from build123d import *

# Parameters (mm, degrees)
SKETCH_2_R          = 10
EXTRUDE_1_DEPTH     = 30
EXTRUDE_START       = -10
EXTRUDE_2_DEPTH     = 10
CUT_EXTRUDE_4_DEPTH = 41.372064023
CUT_EXTRUDE_5_DEPTH = 41.372064023
CUT_EXTRUDE_6_DEPTH = 41.372064023
CUT_EXTRUDE_7_DEPTH = 41.372064023
SKETCH_10_R         = 5.05
CUT_EXTRUDE_8_DEPTH = 25
EXTRUDE_3_DEPTH     = 45
SKETCH_12_R         = 1
CUT_EXTRUDE_9_DEPTH = 79.386948681


with BuildPart() as part:
    # Sketch 2 → Extrude 1 (new body)
    with BuildSketch(Plane(origin=(0, 0, 0), x_dir=(1, 0, 0), z_dir=(0, 1, 0))):
        with Locations(Location((0, 0, 0), (0, 0, 270))):
            Circle(SKETCH_2_R)
    extrude(amount=EXTRUDE_1_DEPTH)

    # Sketch 4 → Extrude 2 (add)
    with BuildSketch(Plane(origin=(0, 30, 0), x_dir=(1, 0, 0), z_dir=(0, 1, 0)).offset(EXTRUDE_START)):
        with BuildLine():
            Line((7.857286278, -21.821134908), (4.965257474, -8.680219941))
            ThreePointArc((4.965257474, -8.680219941), (2.18360644, -9.758681413), (-0.792400015, -9.968555674))
            Line((-0.792400015, -9.968555674), (2.095178486, -23.089249172))
            Line((2.095178486, -23.089249172), (7.857286278, -21.821134908))
        make_face()
    extrude(amount=EXTRUDE_2_DEPTH)

    # Sketch 6 → Cut-Extrude 4 (cut, through all)
    with BuildSketch(Plane(origin=(2.913802079, 0, -0.641264293), x_dir=(-0.2149346210056599, 0, -0.9766284394247146), z_dir=(0.9766284394247146, 0, -0.2149346210056599))):
        with BuildLine():
            Line((-22.999943781, 25.008760147), (-22.999943781, 20))
            Line((-22.999943781, 20), (-18.179619595, 20))
            ThreePointArc((-18.179619595, 20), (-21.599118817, 21.533015498), (-22.999943781, 25.008760147))
        make_face()
    extrude(amount=-CUT_EXTRUDE_4_DEPTH, mode=Mode.SUBTRACT)

    # Sketch 6_3 → Cut-Extrude 5 (cut, through all)
    with BuildSketch(Plane(origin=(2.913802079, 0, -0.641264293), x_dir=(-0.2149346210056599, 0, -0.9766284394247146), z_dir=(0.9766284394247146, 0, -0.2149346210056599))):
        with BuildLine():
            Line((-22.999943781, 30), (-22.999943781, 25.008760147))
            ThreePointArc((-22.999943781, 25.008760147), (-21.691086809, 28.386338596), (-18.448057419, 30))
            Line((-18.448057419, 30), (-22.999943781, 30))
        make_face()
    extrude(amount=-CUT_EXTRUDE_5_DEPTH, mode=Mode.SUBTRACT)

    # Sketch 6_4 → Cut-Extrude 6 (cut, through all)
    with BuildSketch(Plane(origin=(2.913802079, 0, -0.641264293), x_dir=(-0.2149346210056599, 0, -0.9766284394247146), z_dir=(0.9766284394247146, 0, -0.2149346210056599))):
        with BuildLine():
            Line((-15.437501839, 25.006114345), (-20.537499094, 25.01140595))
            ThreePointArc((-20.537499094, 25.01140595), (-17.990146269, 22.45876152), (-15.437501839, 25.006114345))
        make_face()
    extrude(amount=-CUT_EXTRUDE_6_DEPTH, mode=Mode.SUBTRACT)

    # Sketch 6_5 → Cut-Extrude 7 (cut, through all)
    with BuildSketch(Plane(origin=(2.913802079, 0, -0.641264293), x_dir=(-0.2149346210056599, 0, -0.9766284394247146), z_dir=(0.9766284394247146, 0, -0.2149346210056599))):
        with BuildLine():
            ThreePointArc((-15.437500467, 25.008760147), (-17.986177565, 27.558759804), (-20.537499094, 25.01140595))
            Line((-20.537499094, 25.01140595), (-15.437501839, 25.006114345))
            ThreePointArc((-15.437501839, 25.006114345), (-15.43750081, 25.007437246), (-15.437500467, 25.008760147))
        make_face()
        with BuildLine():
            Line((-15.437501839, 25.006114345), (-20.537499094, 25.01140595))
            ThreePointArc((-20.537499094, 25.01140595), (-17.990146269, 22.45876152), (-15.437501839, 25.006114345))
        make_face()
    extrude(amount=-CUT_EXTRUDE_7_DEPTH, mode=Mode.SUBTRACT)

    # Sketch 10 → Cut-Extrude 8 (cut)
    with BuildSketch(Plane.XZ):
        with Locations(Location((0, 0, 0), (0, 0, 270))):
            Circle(SKETCH_10_R)
    extrude(amount=-CUT_EXTRUDE_8_DEPTH, mode=Mode.SUBTRACT)

    # Sketch 11 → Extrude 3 (add)
    with BuildSketch(Plane(origin=(0, 30, 0), x_dir=(1, 0, 0), z_dir=(0, 1, 0))):
        with BuildLine():
            ThreePointArc((-5.777192328, -8.162355592), (-3.40668102, -9.401836227), (-0.792400015, -9.968555674))
            Line((-0.792400015, -9.968555674), (4.965257474, -8.680219941))
            ThreePointArc((4.965257474, -8.680219941), (7.088707625, -7.053383883), (8.704915655, -4.921833342))
            Line((8.704915655, -4.921833342), (8.235679501, -2.824785976))
            Line((8.235679501, -2.824785976), (-6.246428482, -6.065308226))
            Line((-6.246428482, -6.065308226), (-5.777192328, -8.162355592))
        make_face()
        with BuildLine():
            Line((-5.154625262, -10.944648932), (-0.792400015, -9.968555674))
            ThreePointArc((-0.792400015, -9.968555674), (-3.40668102, -9.401836227), (-5.777192328, -8.162355592))
            Line((-5.777192328, -8.162355592), (-5.154625262, -10.944648932))
        make_face()
        with BuildLine():
            ThreePointArc((8.704915655, -4.921833342), (7.088707625, -7.053383883), (4.965257474, -8.680219941))
            Line((4.965257474, -8.680219941), (9.327482721, -7.704126682))
            Line((9.327482721, -7.704126682), (8.704915655, -4.921833342))
        make_face()
    extrude(amount=EXTRUDE_3_DEPTH)

    # Sketch 12 → Cut-Extrude 9 (cut, through all)
    with BuildSketch(Plane(origin=(2.08642873, 0, 9.324387807), x_dir=(0.975868141278159, 0, -0.21836064397759777), z_dir=(0.21836064397759777, 0, 0.975868141278159))):
        with Locations((0, 72.426081563)):
            Circle(SKETCH_12_R)
        with Locations((0, 68.735454777)):
            Circle(SKETCH_12_R)
    extrude(amount=-CUT_EXTRUDE_9_DEPTH, mode=Mode.SUBTRACT)


solid = part.part
Source: CAD feature listing. Evaluate the final solid. Frame: model axes, mm. A direction names the side the tool comes from. Round coordinates to 2 decimals unless told otherwise and drop trailing zeros. Loops run counter-clockwise (first coordinate to the right, second up) from the corner with the lowest first, then second, coordinate; pieces in that order, holes last.
Q1. Access query for faces 1 (the face through (-4, 30, 10)), 2 (the face through (0.31, 24.93, 14.98)), 3 (the face through (8, 30, 7)), 4 (the face through (3, 30, 14)), 5 (the face through (0, 25, 0)). Directions: +Z, -Z, +X, -X, +Y, -Y. A direction counts if a zero-diameter tool reaches every point of the face in a straight line with its end or side. Return the directions, or none.
Q2. Section D-D, the plane x = -1.75. Return loops of the section in (y, z), plus the area to 3 significant figures.
Q3. First-contact query: P1, Ø9, axis at x = -1, z = -5, coming from the +Y side; P2, Ø12, axis at y = 42.5, z = -4, coming from the -X side; P3, Ø2.5, axis at x = 1.5, z = 15.5, coming from the -Y side; P4, Ø1.5, axis at x = -4, y = 66, coming from the -Z side. Flat tips, straight axial feed; report the tip coordinate or a pass-through.
Q4. Section B-B, the plane z = 0. Return loops of the section in (x, y).
Q5. Mould query, pull axis Z, two halves, no side actions, for faces 6 (the face through (1.1, 52.18, 4.42)), 7 (the face through (6.11, 24.93, 13.88)), 8 (the face through (1, 75, 7)). Classes: pulls with the +Z half, pulls with the -Z half, needs draft (parallel to the pull), parting line crosses it, or undercut.
Q6. Ray query, line 1 (X direction, y = 12.75, z = 0); line 2 (Y direction, x = -5.75, z = -2); line 3 (Y direction, x = 4.5, z = 1). Return the intervals inside material, ascending.
Q7. Section C-C, the plane y = 18. Return loops of the section in (x, z).
Q8. Section A-A, the plane y = 62. Return loops of the section in (x, z).
Solutions:
1. face 1: +Z, -X, -Y
1. face 2: +Z, -X, +Y, -Y
1. face 3: +X, -Y
1. face 4: +Z, +X, +Y
1. face 5: -Y
2. outline: (0, -9.85) - (30, -9.85) - (30, 5.06) - (75, 5.06) - (75, 10.18) - (30, 10.18) - (30, 9.85) - (0, 9.85) - (0, 4.74) - (25, 4.74) - (25, -4.74) - (0, -4.74) - close
2. area: 584 mm2
3. P1: stops at y = 30
3. P2: passes through
3. P3: stops at y = 20
3. P4: stops at z = 5.39
4. outline: (-10, 0) - (-5.05, 0) - (-5.05, 25) - (5.05, 25) - (5.05, 0) - (10, 0) - (10, 30) - (-10, 30) - close
5. face 6: pulls with the -Z half
5. face 7: undercut
5. face 8: needs draft
6. line 1: x = -10 to -5.05, 5.05 to 10
6. line 2: y = 0 to 30
6. line 3: y = 25 to 30
7. outline: circle Ø20 at (0, 0); hole circle Ø10.1 at (0, 0)
8. outline: (-6.25, 6.07) - (8.24, 2.82) - (9.33, 7.7) - (-5.15, 10.94) - close
